Here's how the part is built. I have some questions about the finished solid (model axes, mm). A direction names the side the tool comes from. Round coordinates to 2 decimals unless told otherwise and drop trailing zeros. Write each loop counter-clockwise with the first axis right and the second up, starting at its lowest first coordinate (ties: lowest second). Pieces come first, ordered by that corner, then holes. Notation, with made-up numbers: (87, 1) -> (107, 1) arc R15 ccw to (107, 13) -> close; hole circle Ø10 at (59, 46.25). An arc over 180 degrees is marked (long way). Answer in a Markdown table with one row per item.
from build123d import *

# Parameters (mm, degrees)
BOSS_EXTRUDE1_DEPTH = 50
CHAMFER1_SIZE       = 5
FILLET1_R           = 2.54
CUT_EXTRUDE1_DEPTH  = 50
SKETCH4_R           = 11
CUT_EXTRUDE2_DEPTH  = 3


with BuildPart() as part:
    # Sketch1 → Boss-Extrude1 (new body)
    with BuildSketch(Plane.XY):
        Polygon((-58.93139542, -35.722112977), (-55.93139542, -35.722112977), (-55.93139542, 12.277887023), (-7.93139542, 12.277887023), (-7.93139542, 15.277887023), (-58.93139542, 15.277887023), align=None)
    extrude(amount=BOSS_EXTRUDE1_DEPTH)

    # Chamfer1
    chamfer1_edges = [part.edges().sort_by_distance(p)[0] for p in [
        (-7.93139542, 13.777887023, 50),
        (-7.93139542, 13.777887023, 0),
        (-57.43139542, -35.722112977, 50),
        (-57.43139542, -35.722112977, 0),
    ]]
    chamfer(chamfer1_edges, length=CHAMFER1_SIZE)

    # Fillet1
    fillet1_edges = [part.edges().sort_by_distance(p)[0] for p in [
        (-58.93139542, 15.277887023, 25),
        (-55.93139542, 12.277887023, 25),
    ]]
    fillet(fillet1_edges, radius=FILLET1_R)

    # Sketch3 → Cut-Extrude1 (cut)
    with BuildSketch(Plane(origin=(-55.93139542, 0, 0), x_dir=(0, 0, -1), z_dir=(1, 0, 0))):
        with BuildLine():
            Line((-37.85, 5.127887023), (-37.85, -24.572112977))
            ThreePointArc((-37.85, -24.572112977), (-40, -26.722112977), (-42.15, -24.572112977))
            Line((-42.15, -24.572112977), (-42.15, 5.127887023))
            ThreePointArc((-42.15, 5.127887023), (-40, 7.277887023), (-37.85, 5.127887023))
        make_face()
        with BuildLine():
            Line((-12.15, 5.127887023), (-12.15, -24.572112977))
            ThreePointArc((-12.15, -24.572112977), (-10, -26.722112977), (-7.85, -24.572112977))
            Line((-7.85, -24.572112977), (-7.85, 5.127887023))
            ThreePointArc((-7.85, 5.127887023), (-10, 7.277887023), (-12.15, 5.127887023))
        make_face()
    extrude(amount=-CUT_EXTRUDE1_DEPTH, mode=Mode.SUBTRACT)

    # Sketch4 → Cut-Extrude2 (cut)
    with BuildSketch(Plane(origin=(0, 15.277887023, 0), x_dir=(1, 0, 0), z_dir=(0, 1, 0))):
        with Locations(Location((-28.93139542, -25, 0), (0, 0, 180))):
            Circle(SKETCH4_R)
    extrude(amount=-CUT_EXTRUDE2_DEPTH, mode=Mode.SUBTRACT)


solid = part.part
1) I want a section at D-D, the plane z = 10. List the corners of the cut face in (x, y) for me.
Response:
| item | result |
|---|---|
| outline | (-58.93, -35.72) -> (-55.93, -35.72) -> (-55.93, -26.72) -> (-58.93, -26.72) -> close; (-58.93, 7.28) -> (-55.93, 7.28) -> (-55.93, 9.74) arc R2.54 cw to (-53.39, 12.28) -> (-7.93, 12.28) -> (-7.93, 15.28) -> (-56.39, 15.28) arc R2.54 ccw to (-58.93, 12.74) -> close |
2) I need wall thicknesses on line 1 (Z direction, x = -56, y = -23); line 2 (X direction, y = 5, z = 13); line 3 (Y direction, x = -13, z = 39). Which ranges of each line are inside material? Lowest first, please. Write a range as [from, to].
Response:
| item | result |
|---|---|
| line 1 | z = [0, 7.85], [12.15, 37.85], [42.15, 50] |
| line 2 | x = [-58.93, -55.93] |
| line 3 | y = [12.28, 15.28] |
3) We'd pull the mould along Y, two halves only. Please class faces 1 (the face through (-57.41, -26.72, 39.95)), 2 (the face through (-57.41, 7.277, 9.953)), 3 (the face through (-41, 12.278, 25)), 4 (the face through (-43, 15.278, 25)): +Y half, -Y half, draft (parallel to the pull), parting line (faces both ways), or undercut.
Response:
| item | result |
|---|---|
| face 1 | undercut |
| face 2 | undercut |
| face 3 | -Y half |
| face 4 | +Y half |
4) I want a section at C-C, the plane x = -26. List the corners of the cut face in (y, z) for me.
Response:
| item | result |
|---|---|
| outline | (12.28, 0) -> (15.28, 0) -> (15.28, 14.4) -> (12.28, 14.4) -> close; (12.28, 35.6) -> (15.28, 35.6) -> (15.28, 50) -> (12.28, 50) -> close |
5) Which directions (+Z, -Z, +X, -X, +Y, -Y) give clear straight access to the entire face, cutting with the end or side of a thin tool? Please do faces 5 (the face through (-10.47, 13.76, 47.54)), 6 (the face through (-57, -10, 7.85)), 7 (the face through (-55.931, -13, 25)).
Response:
| item | result |
|---|---|
| face 5 | +Z, +X, +Y, -Y |
| face 6 | +X, -X |
| face 7 | +Z, -Z, +X, -Y |
6) I want a section at A-A, the plane y = -1. List the corners of the cut face in (x, z) for me, and give its area (3 significant figures).
Response:
| item | result |
|---|---|
| outline | (-58.93, 0) -> (-55.93, 0) -> (-55.93, 7.85) -> (-58.93, 7.85) -> close; (-58.93, 12.15) -> (-55.93, 12.15) -> (-55.93, 37.85) -> (-58.93, 37.85) -> close; (-58.93, 42.15) -> (-55.93, 42.15) -> (-55.93, 50) -> (-58.93, 50) -> close |
| area | 124 mm^2 |
7) For pin 1 (17.5 mm diameter, centred on x = -28.93, z = 25, fed in from +Y); pin 2 (8 mm diameter, centred on y = -10.5, z = 13, fed in from +X); pin 3 (22.5 mm diameter, centred on x = -34.5, z = 35, fed in from -Y), each with a flat end and sliding along its axis, tell me the tip position at first contact or that it passes through.
Response:
| item | result |
|---|---|
| pin 1 | passes through |
| pin 2 | stops at x = -55.93 |
| pin 3 | stops at y = 12.28 |
8) I want a section at B-B, the plane z = 25. List the corners of the cut face in (x, y) for me.
Response:
| item | result |
|---|---|
| outline | (-58.93, -35.72) -> (-55.93, -35.72) -> (-55.93, 9.74) arc R2.54 cw to (-53.39, 12.28) -> (-39.93, 12.28) -> (-39.93, 15.28) -> (-56.39, 15.28) arc R2.54 ccw to (-58.93, 12.74) -> close; (-17.93, 12.28) -> (-7.93, 12.28) -> (-7.93, 15.28) -> (-17.93, 15.28) -> close |
